```python
from build123d import *

# Parameters (mm, degrees)
F1_DEPTH = 603.25
F3_R     = 3.175
F4_DEPTH = 50.8
F5_DEPTH = 50.8
F6_R     = 3.175
F7_DEPTH = 6.35


with BuildPart() as f1:
    # F0 (on Front) → F1 (new body, symmetric)
    with BuildSketch(Plane.XZ):
        Polygon((-19.05, -31.75), (19.05, -31.75), (19.05, 31.75), (11.1125, 31.75), (11.1125, 21.59), (7.9375, 21.59), (7.9375, 31.75), (-7.9375, 31.75), (-7.9375, 21.59), (-11.1125, 21.59), (-11.1125, 31.75), (-19.05, 31.75), align=None)
    extrude(amount=F1_DEPTH, both=True)

    # F3 (on face) → F4 (cut)
    with BuildSketch(Plane.XY.offset(31.75)):
        with Locations((0, 574.675)):
            Circle(F3_R)
        with Locations((0, -574.675)):
            Circle(F3_R)
    extrude(amount=-F4_DEPTH, mode=Mode.SUBTRACT)

    # F2 (on face) → F5 (cut)
    with BuildSketch(Plane.YZ.offset(19.05)):
        Polygon((603.25, 31.75), (539.75, 31.75), (603.25, -31.75), align=None)
        Polygon((-603.25, 31.75), (-603.25, -31.75), (-539.75, 31.75), align=None)
    extrude(amount=-F5_DEPTH, mode=Mode.SUBTRACT)

    # F6 (on face) → F7 (cut)
    with BuildSketch(Plane(origin=(0, 0, -31.75), x_dir=(1, 0, 0), z_dir=(0, 0, -1))):
        with Locations((0, -457.2)):
            Circle(F6_R)
        with Locations((0, -152.4)):
            Circle(F6_R)
        with Locations((0, 152.4)):
            Circle(F6_R)
        with Locations((0, 457.2)):
            Circle(F6_R)
    extrude(amount=-F7_DEPTH, mode=Mode.SUBTRACT)


solid = f1.part
```
Geometry check sheet. Reference: the model listing, model coordinates, mm. Coordinates: 2 decimals unless noted, no trailing zeros. Loops run counter-clockwise (first coordinate to the right, second up) from the corner with the lowest first, then second, coordinate; pieces in that order, holes last. Notation, with made-up numbers: (37.5, -37.75) -> (82.5, -37.75) arc R32 cw to (82.5, -9.75) -> close; hole circle Ø9 at (14, 31.5). An arc over 180 degrees is marked (long way). Put each result on its own line as item: value.
1) Cross-section at A-A on y = 42. Record the boundary of the cut face in (x, z).
Result set:
outline: (-19.05, -31.75) -> (19.05, -31.75) -> (19.05, 31.75) -> (11.11, 31.75) -> (11.11, 21.59) -> (7.94, 21.59) -> (7.94, 31.75) -> (-7.94, 31.75) -> (-7.94, 21.59) -> (-11.11, 21.59) -> (-11.11, 31.75) -> (-19.05, 31.75) -> close
2) Gauge pin test, flat ends, axial feed: pin 1 Ø5 at (x, y) = (0, 152.4) entering from -Z; pin 2 Ø4 at (x, z) = (-11.5, 3.5) entering from -Y; pin 3 Ø8.5 at (x, y) = (0, -457.2) entering from -Z; pin 4 Ø10 at (x, z) = (2.5, -6.5) entering from +Y. Record the tip position at first contact, or that the pin passes through.
Result set:
pin 1: stops at z = -25.4
pin 2: stops at y = -570
pin 3: stops at z = -31.75
pin 4: stops at y = 583
3) Thickness scan on line 1 (X direction, y = 348, z = 26.5); line 2 (Y direction, x = 0, z = -29) (3 decimals); line 3 (X direction, y = 152, z = -27). Record the ranges inside material, lowest first.
Result set:
line 1: x = -19.05 to -11.11, -7.94 to 7.94, 11.11 to 19.05
line 2: y = -600.5 to -460.375, -454.025 to -155.575, -149.225 to 149.225, 155.575 to 454.025, 460.375 to 600.5
line 3: x = -19.05 to -3.15, 3.15 to 19.05
